Here's how the part is built. I have some questions about the finished solid (model axes, mm). Face numbers are marked on the shaded views. A direction names the side the tool comes from. Round coordinates to 2 decimals unless told otherwise and drop trailing zeros. Order: outer loops, then holes, each group sorted by start corner. A loop starts at its lowest first (then second) coordinate and runs counter-clockwise, first axis right, second up. Notation, with made-up numbers: (43.5, 71) -> (82.5, 71) arc R22 ccw to (82.5, 80) -> close; hole circle Ø8 at (-35.5, 57). An arc over 180 degrees is marked (long way). Use a Markdown table: item, result. Add a question column.
(1) On a 3-axis mill with a long thin cutter (end or side, diameter ignored), from which of +Z, -Z, +X, -X, +Y, -Y can I reach the whole of each face in a straight line? I mean the marked faces 1, 2 and 3. Say none if no direction works.
(2) I want a section at B-B, the plane y = 2.5. Please give me the cut outline in (x, z).
(3) If I drill on probe 1 along Y at (x, z) = (-2, -2); probe 2 along Z at (x, y) = (-1, -11.75); probe 3 along Z at (x, y) = (-0.25, 3.25), over which ranges is the centre line in solid material (lowest first)?
(4) Thinking about a two-plate mould opening in Z: for the marked faces 4, 5 and 6, which applies, pulls with the +Z half, pulls with the -Z half, needs draft (parallel to the pull), parting line crosses it, or undercut?
(5) I'm going to push flat-ended pins straight in: P1, Ø4, axis at x = 2.5, y = -5.5, coming from the -Z side; P2, Ø1.5, axis at x = 0.5, y = -10.5, coming from the -Z side; P3, Ø2, axis at x = -1, y = -14, coming from the +Z side; P4, Ø2.5, axis at x = 0, z = 0.5, coming from the +Y side. Where does each tip first touch, or does it pass through?
(6) I want a section at D-D, the plane y = -11.5. Please give me the cut outline in (x, z).
(7) I want a section at C-C, the plane x = -0.75. Please give me the cut outline in (y, z), then the cut area to 3 significant figures.
(8) I want a section at A-A, the plane z = 0. Please give me the cut outline in (x, y).
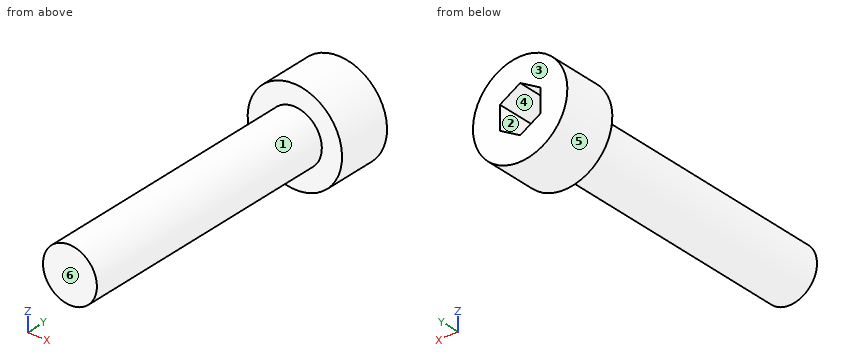
from build123d import *

# Parameters (mm, degrees)
SKETCH2_R           = 3.5
BOSS_EXTRUDE1_DEPTH = 4
SKETCH3_R           = 2
BOSS_EXTRUDE2_DEPTH = 20


with BuildPart() as part:
    # Sketch2 → Boss-Extrude1 (new body)
    with BuildSketch(Plane(origin=(0, 0, 0), x_dir=(1, 0, 0), z_dir=(0, 1, 0))):
        with Locations(Location((0, 0, 0), (0, 0, 270))):
            Circle(SKETCH2_R)
        Polygon((0, 1.732050808), (-1.5, 0.866025404), (-1.5, -0.866025404), (0, -1.732050808), (1.5, -0.866025404), (1.5, 0.866025404), align=None, mode=Mode.SUBTRACT)
    extrude(amount=BOSS_EXTRUDE1_DEPTH)

    # Sketch3 → Boss-Extrude2 (add)
    with BuildSketch(Plane.XZ):
        with Locations(Location((0, 0, 0), (0, 0, 90))):
            Circle(SKETCH3_R)
    extrude(amount=BOSS_EXTRUDE2_DEPTH)


solid = part.part
Taken from the geometry:
| question | item | result |
|---|---|---|
| 1 | face 1 | -Y |
| 1 | face 2 | +Y |
| 1 | face 3 | +Z, -Z, +X, -X, +Y |
| 2 | outline | circle Ø7 at (0, 0); hole (-1.5, -0.87) -> (0, -1.73) -> (1.5, -0.87) -> (1.5, 0.87) -> (0, 1.73) -> (-1.5, 0.87) -> close |
| 3 | probe 1 | y = 0 to 4 |
| 3 | probe 2 | z = -1.73 to 1.73 |
| 3 | probe 3 | z = -3.49 to -1.59, 1.59 to 3.49 |
| 4 | face 4 | undercut |
| 4 | face 5 | parting line crosses it |
| 4 | face 6 | needs draft |
| 5 | P1 | stops at z = -1.94 |
| 5 | P2 | stops at z = -2 |
| 5 | P3 | stops at z = 2 |
| 5 | P4 | stops at y = 4 |
| 6 | outline | circle Ø4 at (0, 0) |
| 7 | outline | (-20, -1.85) -> (0, -1.85) -> (0, -3.42) -> (4, -3.42) -> (4, -1.3) -> (0, -1.3) -> (0, 1.3) -> (4, 1.3) -> (4, 3.42) -> (0, 3.42) -> (0, 1.85) -> (-20, 1.85) -> close |
| 7 | area | 91.1 mm2 |
| 8 | outline | (-3.5, 0) -> (-2, 0) -> (-2, -20) -> (2, -20) -> (2, 0) -> (3.5, 0) -> (3.5, 4) -> (1.5, 4) -> (1.5, 0) -> (-1.5, 0) -> (-1.5, 4) -> (-3.5, 4) -> close |
